Geometry check sheet. Reference: the model listing, model coordinates, mm. A direction names the side the tool comes from. Coordinates: 2 decimals unless noted, no trailing zeros. Loops run counter-clockwise (first coordinate to the right, second up) from the corner with the lowest first, then second, coordinate; pieces in that order, holes last. Notation, with made-up numbers: (87.5, -34.75) - (118.5, -34.75) arc R14 cw to (118.5, -17.75) - close; hole circle Ø10 at (15, 11.5). An arc over 180 degrees is marked (long way). Write item = value, one per line. Start each with the question number.
from build123d import *

# Parameters (mm, degrees)
CYLINDER_R     = 1.8
CYLINDER_DEPTH = 40
PAD_DEPTH      = 10


with BuildPart() as hole:
    # Cylinder → Cylinder (new body)
    with BuildSketch(Plane(origin=(-25, -5, -8), x_dir=(0, 0, -1), z_dir=(1, 0, 0))):
        Circle(CYLINDER_R)
    extrude(amount=CYLINDER_DEPTH)


with BuildPart() as cut:
    # Sketch → Pad (new body)
    with BuildSketch(Plane.XZ):
        with BuildLine():
            Line((-7.5, -13), (-7.5, 20))
            Line((-7.5, 20), (-5.5, 20))
            add(Edge.make_bspline(
                [(-5.5, 20), (-5.5, 1.17), (0, 0), (5.5, 1.17), (5.5, 6)],
                knots=[0, 0, 0, 0, 0.5, 1, 1, 1, 1], degree=3))
            Line((5.5, 6), (7.5, 6))
            Line((7.5, 6), (7.5, -3))
            Line((7.5, -3), (-3.5, -3))
            Line((-3.5, -3), (-3.5, -13))
            Line((-3.5, -13), (-7.5, -13))
        make_face()
    extrude(amount=PAD_DEPTH)

    # Cut: cut hole
    add(hole.part, mode=Mode.SUBTRACT)


solid = cut.part
(1) Depth check by flat-ended pin: pin 1 (2 mm diameter, centred on x = 6.5, y = -6, fed in from +Z); pin 2 (2 mm diameter, centred on y = -5, z = -8, fed in from +X); pin 3 (5 mm diameter, centred on y = -6.5, z = -6, fed in from +X). Enter the tip coordinate at first touch or a pass-through.
(2) Sectioned sample at A-A on z = -8. Enter the section's corners in (x, y).
(3) Draft check along Z on faces 4 (the face through (-5.528, -3.783, -6.673)), 5 (the face through (2, -5, -3)), 6 (the face through (-3, -10, 1)). Enter one of: pulls with the +Z half, pulls with the -Z half, needs draft (parallel to the pull), parting line crosses it, or undercut.
(4) Tool access check on faces 1 (the face through (-7.5, -5, 3)), 2 (the face through (-3.5, -5, -10)), 3 (the face through (6, -5, 6)). Record the directions out of +Z, -Z, +X, -X, +Y, -Y that give a thin tool (end or side, any length) a straight path to the whole face; none if there is none.
(5) Scan lines: line 1 (Y direction, x = -5.2, z = -8); line 2 (Z direction, x = -5.95, y = -5); line 3 (X direction, y = -7.5, z = -6). Record each from-to range of solid material in increasing order.
Working result:
q1.pin_1 = 6
q1.pin_2 = through
q1.pin_3 = -3.5
q2.outline = (-7.5, -10) - (-3.5, -10) - (-3.5, -6.8) - (-7.5, -6.8) - close; (-7.5, -3.2) - (-3.5, -3.2) - (-3.5, 0) - (-7.5, 0) - close
q3.face_4 = undercut
q3.face_5 = pulls with the -Z half
q3.face_6 = needs draft
q4.face_1 = +Z, -Z, -X, +Y, -Y
q4.face_2 = -Z, +X, +Y, -Y
q4.face_3 = +Z, +X, +Y, -Y
q5.line_1 = -10 to -6.8, -3.2 to 0
q5.line_2 = -13 to -9.8, -6.2 to 20
q5.line_3 = -7.5 to -3.5
